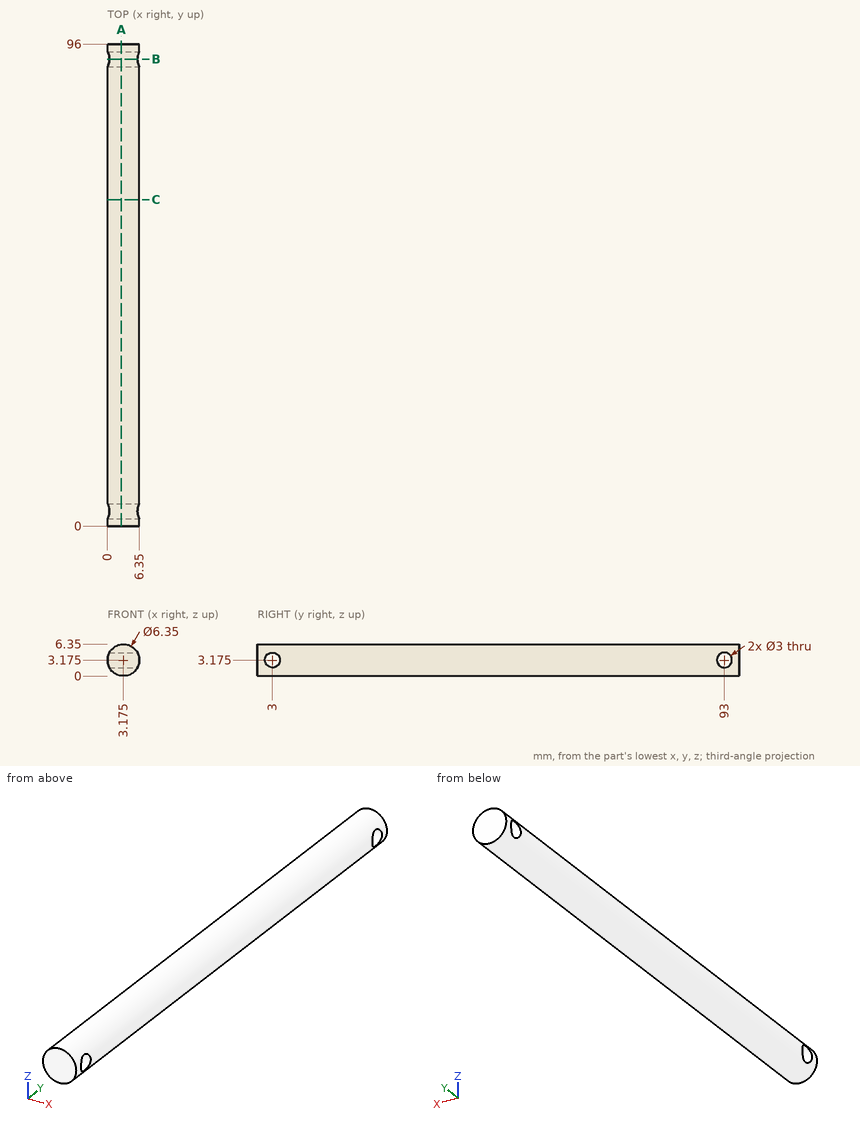
Drawing for the job (mm, zero at the part's lowest x, y, z). Round coordinates to 2 decimals unless told otherwise and drop trailing zeros. Write each loop counter-clockwise with the first axis right and the second up, starting at its lowest first coordinate (ties: lowest second). Pieces come first, ordered by that corner, then holes. Notation, with made-up numbers: M -15.75,-24 L -2.75,-24 A17 ccw -2.75,-16 Z; hole C -6.5,-23 d8. An arc over 180 degrees is marked long. Answer as a JSON object with one key per item and string values. Group by question number.
(1) Cut at A-A (x = 2.75). Give the cut face in (y, z) (3 decimals).
(2) Flat gauge pins, fed straight in: pin 1 (2.5 mm diameter, centred on y = 93, z = 3.175, fed in from -X); pin 2 (1 mm diameter, centred on y = 69, z = 5, fed in from +X). Where does each tip first touch, or does it go through?
(3) Drill centre lines: L1, parallel to Y at x = 1, z = 3.25; L2, parallel to Y at x = 4.5, z = 2.25; L3, parallel to Z at x = 3.25, y = 65.5. Where is each one in solid material? Low to high.
(4) Cut at B-B (y = 93). Give the cut face in (x, z) (3 decimals).
(5) Cut at C-C (y = 65). Give the cut face in (x, z) (3 decimals).
Responses:
{
 "1": {"outline": "M 0,0.029 L 96,0.029 L 96,6.321 L 0,6.321 Z; hole C 3,3.175 d3; hole C 93,3.175 d3"},
 "2": {"pin 1": "passes through", "pin 2": "stops at x = 6.06"},
 "3": {"L1": "y = 0 to 1.5, 4.5 to 91.5, 94.5 to 96", "L2": "y = 0 to 1.82, 4.18 to 91.82, 94.18 to 96", "L3": "z = 0 to 6.35"},
 "4": {"outline": "M 0.377,1.675 A3.175 ccw 5.973,1.675 Z; M 0.377,4.675 L 5.973,4.675 A3.175 ccw Z"},
 "5": {"outline": "C 3.175,3.175 d6.35"}
}
